Verification items for this drawing (mm, ordinates from the low corner). A direction names the side the tool comes from. Coordinates: 2 decimals unless noted, no trailing zeros. Write each loop counter-clockwise with the first axis right and the second up, starting at its lowest first coordinate (ties: lowest second). Pieces come first, ordered by that corner, then holes. Notation, with made-up numbers: (4, -9.75) -> (42, -9.75) arc R12 cw to (42, 4.25) -> close; hole circle Ø1 at (84, 30). An arc over 180 degrees is marked (long way). Use CSV: the item, a comma, the result in double quotes.
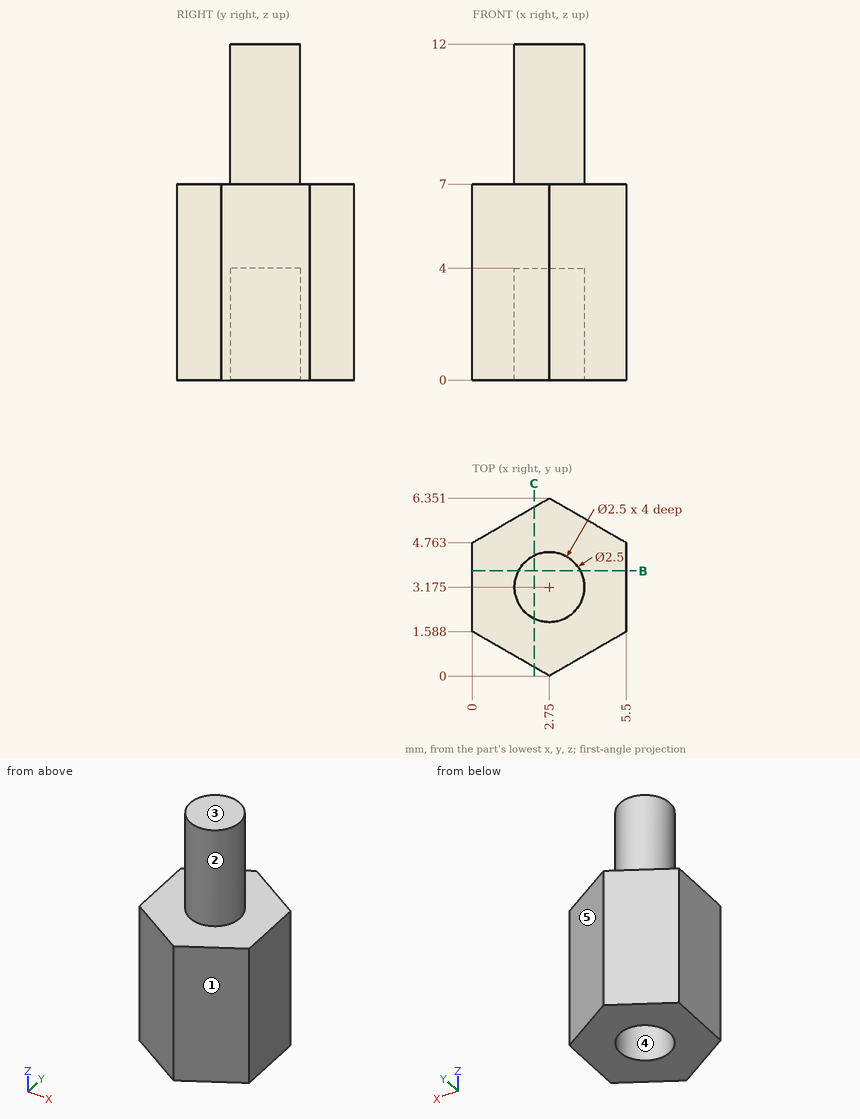
1) Cross-section at C-C (x = 2.2). Record the boundary of the cut face in (y, z).
Return value:
outline,"(0.32, 0) -> (2.05, 0) -> (2.05, 4) -> (4.3, 4) -> (4.3, 0) -> (6.03, 0) -> (6.03, 7) -> (4.3, 7) -> (4.3, 12) -> (2.05, 12) -> (2.05, 7) -> (0.32, 7) -> close"
2) Gauge pin test, flat ends, axial feed: pin 1 (1.5 mm diameter, centred on y = 2.5, z = 8, fed in from +X); pin 2 (1.2 mm diameter, centred on x = 2.5, y = 3.5, fed in from -Z). Record the tip position at first contact, or that the pin passes through.
Return value:
pin 1,"x = 4"
pin 2,"z = 4"
3) Mould release check, pull along Y, two halves, no side actions. Record for the marked faces 3, 4 and 5: released by +Y, released by -Y, zero draft, split by the parting line, or undercut.
Return value:
face 3,"zero draft"
face 4,"undercut"
face 5,"released by +Y"
4) Cross-section at B-B (y = 3.75). Record the boundary of the cut face in (x, z).
Return value:
outline,"(0, 0) -> (1.64, 0) -> (1.64, 4) -> (3.86, 4) -> (3.86, 0) -> (5.5, 0) -> (5.5, 7) -> (3.86, 7) -> (3.86, 12) -> (1.64, 12) -> (1.64, 7) -> (0, 7) -> close"
5) Scan lines: L1, parallel to Z at x = 5.15, y = 4.75; L2, parallel to X at y = 3.25, z = 0.75; L3, parallel to Y at x = 3.2, z = 3.25. Record each from-to range of solid material in increasing order.
Return value:
L1,"0 to 7"
L2,"0 to 1.5, 4 to 5.5"
L3,"0.26 to 2.01, 4.34 to 6.09"
6) Set-up check for the marked faces 1 and 2: record each of +Z, -Z, +X, -X, +Y, -Y from which the full face is reachable in a straight line by a thin tool's end or side.
Return value:
face 1,"+Z, -Z, +X, -Y"
face 2,"+Z"
